Could you check a few things on this model? Use its own coordinates, in mm. Face numbers are marked on the shaded views. Give positions to 0.01 mm unless a question says otherwise; leave off trailing zeros. Loops run counter-clockwise (first coordinate to the right, second up) from the corner with the lowest first, then second, coordinate; pieces in that order, holes last. Notation, with made-up numbers: M -14.5,-16 L -8.5,-16 A10 cw -8.5,-7 Z; hole C 51.5,23.5 d9. An arc over 180 degrees is marked long. Write each question's results on one line, items separated by ' | '. Start each with the question number.
Autodesk Inventor part; units mm, degrees
ref_plane "YZ Plane" through (0, 0, 0) normal (1, 0, 0) x (0, 1, 0)
ref_plane "XZ Plane" through (0, 0, 0) normal (0, 1, 0) x (-1, 0, 0)
ref_plane "XY Plane" through (0, 0, 0) normal (0, 0, 1) x (1, 0, 0)
sketch "Sketch1" plane through (0, 0, 0) normal (1, 0, 0) x (0, 1, 0)
  circle A0 centre (0, 0) radius 4
  circle A1 centre (0, 0) radius 13
  dimension "d0" = 8
  dimension "d1" = 26
extrude "Extrusion1" add sketch "Sketch1" along normal blind 2.5
sketch "Sketch2" plane through (2.5, 0, 0) normal (1, 0, 0) x (0, 0, -1)
  circle A0 centre (0, 0) radius 3
  circle A1 centre (0, 0) radius 13
  dimension "d4" = 6
extrude "Extrusion2" add sketch "Sketch2" along normal blind 5.5
sketch "Sketch3" plane through (8, 0, 0) normal (1, 0, 0) x (0, 0, -1)
  circle A0 centre (0, 0) radius 3
  circle A1 centre (0, 0) radius 11.08
  dimension "d7" = 22.16
extrude "Extrusion3" add sketch "Sketch3" along normal blind 16
sketch "Sketch4" plane through (24, 0, 0) normal (1, 0, 0) x (0, 0, -1)
  circle A0 centre (0, 0) radius 13
  circle A1 centre (0, 0) radius 3
extrude "Extrusion4" add sketch "Sketch4" along normal blind 1
sketch "Sketch5" plane through (25, 0, 0) normal (1, 0, 0) x (0, 0, -1)
  circle A0 centre (0, 0) radius 4
  dimension "d12" = 8
extrude "Extrusion5" cut sketch "Sketch5" against normal blind 2.5
chamfer "Chamfer1" distance 2.5 angle 2 1 edges at (0, -4, 0) measured on face at (1.6667, 3.9482, -0.6416)
chamfer "Chamfer2" distance 2.5 angle 2 1 edges at (25, 0, 4) measured on face at (23.3333, -0.6416, -3.9482)
sketch "Sketch6" plane through (0, 0, 0) normal (-1, 0, 0) x (0, 0, 1)
  line L0 (0.2, 4.0824) -> (0.2, 3.995)
  line L1 (-0.2, 4.0824) -> (-0.2, 3.995)
  line L2 (0, 0) -> (0, 3.9651) construction
  circle A0 centre (0, 0) radius 4 construction
  arc A1 (-0.2, 4) -> (0.2, 4) centre (0, 4) ccw
  circle A2 centre (0, 0) radius 4.0873
  line L3 (-3.4355, -2.2144) -> (-3.3598, -2.1707)
  arc A3 (-3.3641, -2.1732) -> (-3.5641, -1.8268) centre (-3.4641, -2) ccw
  line L4 (-3.6355, -1.868) -> (-3.5598, -1.8243)
  line L5 (3.6355, -1.868) -> (3.5598, -1.8243)
  arc A4 (3.5641, -1.8268) -> (3.3641, -2.1732) centre (3.4641, -2) ccw
  line L6 (3.4355, -2.2144) -> (3.3598, -2.1707)
  dimension "d21" = 0.2
  dimension "d22" = 0.2
  dimension "d23" = 0.4
  dimension "d26" = 360
extrude "Extrusion6" add sketch "Sketch6" against normal blind 2.5 contours L0 A1 L1 A2 | A2 L6 A4 L5 | L4 A3 L3 A2
sketch "Sketch7" plane through (25, 0, 0) normal (1, 0, 0) x (0, 0, -1)
  circle A0 centre (0, 0) radius 13
  arc A1 (-0.2, 4.0824) -> (-3.6355, -1.868) centre (0, 0) ccw
  line L0 (-3.6355, -1.868) -> (-3.5641, -1.8268)
  arc A2 (-3.3641, -2.1732) -> (-3.5641, -1.8268) centre (-3.4641, -2) ccw
  line L1 (-3.3641, -2.1732) -> (-3.4355, -2.2144)
  arc A3 (-3.4355, -2.2144) -> (3.4355, -2.2144) centre (0, 0) ccw
  line L2 (3.4355, -2.2144) -> (3.3641, -2.1732)
  arc A4 (3.5641, -1.8268) -> (3.3641, -2.1732) centre (3.4641, -2) ccw
  line L3 (3.5641, -1.8268) -> (3.6355, -1.868)
  arc A5 (3.6355, -1.868) -> (0.2, 4.0824) centre (0, 0) ccw
  line L4 (0.2, 4.0824) -> (0.2, 4)
  arc A6 (-0.2, 4) -> (0.2, 4) centre (0, 4) ccw
  line L5 (-0.2, 4) -> (-0.2, 4.0824)
  circle A7 centre (0, 0) radius 13
  circle A8 centre (0, 0) radius 4.0873
  point P0 (3.4355, -2.2144)
  point P1 (-3.6355, -1.868)
  point P2 (0.2, 4.0824)
  point P3 (-0.2, 4.0824)
extrude "Extrusion7" add sketch "Sketch7" against normal blind 2.5 contours A8 L4 A6 L5 | L0 A2 L1 A8 | L2 A4 L3 A8
fillet "Fillet1" radius 0.6 6 edges at (25, 2.0434, -3.5393) (25, -4.0868, 0) (25, 2.0434, 3.5393) (0, 2.0434, -3.5393) (0, 2.0434, 3.5393) (0, -4.0868, 0)
properties part number "8mm ID 15mm Deep Idler Pully"
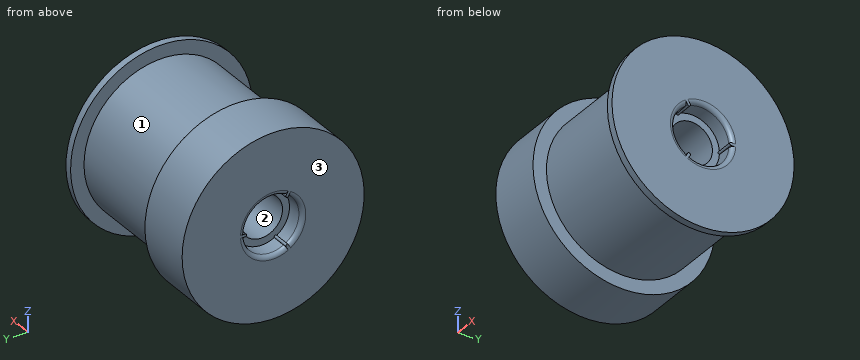
1) If we section it at D-D on y = -10: Write out the boundary of the cut face in (x, z).
2) Thinking about a two-plate mould opening in Y: for the marked faces 1, 2 and 3, which applies, pulls with the +Y half, pulls with the -Y half, needs draft (parallel to the pull), parting line crosses it, or undercut?
3) If we section it at B-B on x = 19.25: Write out the boundary of the cut face in (y, z), plus the area to 3 significant figures.
4) If we section it at C-C on z = -7.75: Write out the boundary of the cut face in (x, y).
5) I'm going to push flat-ended pins straight in: P1, Ø6, axis at x = 3, z = -9, coming from the -Y side; P2, Ø7, axis at y = 0, z = 0, coming from the -X side; P3, Ø8, axis at x = 3.5, y = -8, coming from the -Z side. Where does each tip first touch, or does it pass through?
6) Please list where these lines run through material, in increasing order: line 1 (Y direction, x = 17.5, z = 0); line 2 (X direction, y = 9.75, z = 7.75); line 3 (X direction, y = -3, z = 3.5). Write a range as from..to.
Calculated:
1) outline: M 0,-8.31 L 8,-8.31 L 8,-4.77 L 24,-4.77 L 24,-8.31 L 25,-8.31 L 25,8.31 L 24,8.31 L 24,4.77 L 8,4.77 L 8,8.31 L 0,8.31 Z
2) face 1: parting line crosses it | face 2: undercut | face 3: needs draft
3) outline: C 0,0 d22.16; hole C 0,0 d6 | area: 357 mm2
4) outline: M 0,-10.44 L 8,-10.44 L 8,-7.92 L 24,-7.92 L 24,-10.44 L 25,-10.44 L 25,10.44 L 24,10.44 L 24,7.92 L 8,7.92 L 8,10.44 L 0,10.44 Z
5) P1: stops at y = -11.53 | P2: stops at x = 2.5 | P3: stops at z = -12.37
6) line 1: y = -11.08..-3, 3..11.08 | line 2: x = 0..8, 24..25 | line 3: x = 0..25
